Design review of the part built by this model. Coordinates are the model's own, in mm. Give positions to 0.01 mm unless a question says otherwise; leave off trailing zeros. Order: outer loops, then holes, each group sorted by start corner. A loop starts at its lowest first (then second) coordinate and runs counter-clockwise, first axis right, second up. Notation, with made-up numbers: (25.5, 37) -> (43.5, 37) arc R25 cw to (43.5, 64) -> close; hole circle Ø2 at (32, -10). An arc over 180 degrees is marked (long way). Return JSON: item names as keys, results as strings.
```python
from build123d import *

# Parameters (mm, degrees)
SKETCH1_W           = 20
SKETCH1_H           = 20
BOSS_EXTRUDE1_DEPTH = 10
CUT_EXTRUDE1_DEPTH  = 21
CUT_EXTRUDE2_DEPTH  = 21


with BuildPart() as part:
    # Sketch1 → Boss-Extrude1 (new body)
    with BuildSketch(Plane(origin=(0, 0, 0), x_dir=(1, 0, 0), z_dir=(0, 1, 0))):
        with Locations((10, 10)):
            Rectangle(SKETCH1_W, SKETCH1_H)
    extrude(amount=BOSS_EXTRUDE1_DEPTH)

    # Sketch2 → Cut-Extrude1 (cut, through all)
    with BuildSketch(Plane(origin=(20, 0, 0), x_dir=(0, 0, -1), z_dir=(1, 0, 0))):
        Polygon((20, 1.5), (11.5, 10), (20, 10), align=None)
        with BuildLine():
            Line((0, 1.5), (0, 10))
            Line((0, 10), (8.5, 10))
            ThreePointArc((8.5, 10), (2.48959236, 7.51040764), (0, 1.5))
        make_face()
    extrude(amount=-CUT_EXTRUDE1_DEPTH, mode=Mode.SUBTRACT)

    # Sketch3 → Cut-Extrude2 (cut, through all)
    with BuildSketch(Plane(origin=(0, 0, -20), x_dir=(-1, 0, 0), z_dir=(0, 0, -1))):
        Polygon((-20, 0), (-10, 10), (-20, 10), align=None)
    extrude(amount=-CUT_EXTRUDE2_DEPTH, mode=Mode.SUBTRACT)


solid = part.part
```
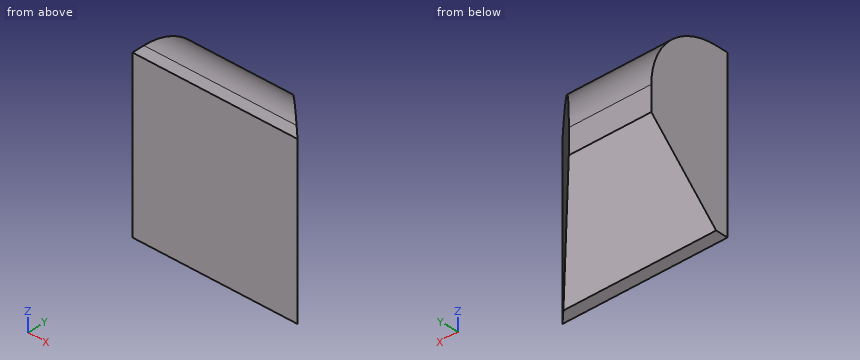
Item 1: Add section B-B (x = 7). Give the boundary of the cut face in (y, z), plus the area to 3 significant figures.
Result set:
{"outline": "(0, -20) -> (1.5, -20) -> (10, -11.5) -> (10, -8.5) arc R8.5 ccw to (1.5, 0) -> (0, 0) -> close", "area": "148 mm^2"}
Item 2: Add section A-A (z = -13). Give the boundary of the cut face in (x, y).
Result set:
{"outline": "(0, 0) -> (20, 0) -> (11.5, 8.5) -> (0, 8.5) -> close"}
Item 3: For pin 1 (3 mm diameter, centred on x = 13.5, z = -9.5, fed in from +Y); pin 2 (8 mm diameter, centred on x = 17.5, z = -7.5, fed in from +Y); pin 3 (6 mm diameter, centred on x = 4.5, y = 6.5, fed in from -Z), all flat-tipped, find the tip position at first contact; note any pin that passes through.
Result set:
{"pin 1": "stops at y = 8", "pin 2": "stops at y = 6.5", "pin 3": "stops at z = -18"}
Item 4: Wall thickness on L1, parallel to X at y = 4, z = -7.5; L2, parallel to X at y = 4.75, z = -8.75; L3, parallel to Z at x = 3, y = 5.5: over which ranges is each line inside the solid? List them lowest first. Write a range as [from, to].
Result set:
{"L1": "x = [0, 16]", "L2": "x = [0, 15.25]", "L3": "z = [-16, -1]"}
Item 5: Add section C-C (y = 6). Give the boundary of the cut face in (x, z), plus the area to 3 significant figures.
Result set:
{"outline": "(0, -15.5) -> (14, -15.5) -> (14, -1.29) -> (0, -1.29) -> close", "area": "199 mm^2"}
Item 6: Add section D-D (x = 12.5). Give the boundary of the cut face in (y, z), plus the area to 3 significant figures.
Result set:
{"outline": "(0, -20) -> (1.5, -20) -> (7.5, -14) -> (7.5, -2.48) arc R8.5 ccw to (1.5, 0) -> (0, 0) -> close", "area": "127 mm^2"}
